```python
from build123d import *
from build123d.topology import SkipClean

# Parameters (mm, degrees)
SKETCH1_W               = 15
SKETCH1_H               = 23.93877551
BOSS_EXTRUDE1_DEPTH     = 25
CUT_EXTRUDE1_DEPTH      = 25
CUT_EXTRUDE2_DEPTH      = 33.787192622
CUT_EXTRUDE2_DEPTH_BACK = 33.787192622
SKETCH3_R               = 2.75
SKETCH4_W               = 9.5
SKETCH4_H               = 17
CUT_EXTRUDE3_DEPTH      = 8
CHAMFER1_SIZE           = 2
BOSS_EXTRUDE2_DEPTH     = 12.7
CHAMFER2_START          = 15.513056934
CHAMFER2_OUTLINE_W      = 15
CHAMFER2_OUTLINE_H      = 24
CHAMFER2_DEPTH          = 11.486943066


with BuildPart() as part:
    # Sketch1 → Boss-Extrude1 (new body)
    with BuildSketch(Plane.XY):
        with Locations((7.5, 11.969387755)):
            Rectangle(SKETCH1_W, SKETCH1_H)
    extrude(amount=BOSS_EXTRUDE1_DEPTH)

    # Sketch2 → Cut-Extrude1 (cut)
    with BuildSketch(Plane.XY.offset(25)):
        with BuildLine():
            Line((0, 8.93877551), (0, 0))
            Line((0, 0), (15, 0))
            Line((15, 0), (15, 8.93877551))
            ThreePointArc((15, 8.93877551), (7.5, 9.487151408), (0, 8.93877551))
        make_face()
    extrude(amount=-CUT_EXTRUDE1_DEPTH, mode=Mode.SUBTRACT)

    # Sketch3 → Cut-Extrude2 (cut, two sides: drawn at the far end of the back side and taken through both)
    with BuildSketch(Plane(origin=(0, 23.93877551, 0), x_dir=(1, 0, 0), z_dir=(0, 1, 0)).offset(-CUT_EXTRUDE2_DEPTH_BACK)):
        with Locations(Location((7.5, -8.825, 0), (0, 0, 270))):
            Circle(SKETCH3_R)
        with Locations(Location((7.5, -16.175, 0), (0, 0, 270))):
            Circle(SKETCH3_R)
    extrude(amount=CUT_EXTRUDE2_DEPTH + CUT_EXTRUDE2_DEPTH_BACK, mode=Mode.SUBTRACT)

    # Sketch4 → Cut-Extrude3 (cut)
    with BuildSketch(Plane(origin=(0, 23.93877551, 0), x_dir=(1, 0, 0), z_dir=(0, 1, 0))):
        with Locations((7.5, -12.5)):
            Rectangle(SKETCH4_W, SKETCH4_H)
    extrude(amount=-CUT_EXTRUDE3_DEPTH, mode=Mode.SUBTRACT)

    # Chamfer1
    chamfer1_edges = [part.edges().sort_by_distance(p)[0] for p in [
        (2.75, 19.93877551, 4),
        (12.25, 19.93877551, 4),
    ]]
    chamfer(chamfer1_edges, length=CHAMFER1_SIZE)

    # Sketch5 → Boss-Extrude2 (add)
    with SkipClean():  # the faces are left unmerged after this step: merging them gives an invalid solid
        with BuildSketch(Plane(origin=(0, 0, 0), x_dir=(-1, 0, 0), z_dir=(0, 0, -1))):
            with BuildLine():
                Line((-15, 23.93877551), (0, 23.93877551))
                Line((0, 23.93877551), (0, 8.93877551))
                ThreePointArc((0, 8.93877551), (-7.5, 9.487151408), (-15, 8.93877551))
                Line((-15, 8.93877551), (-15, 23.93877551))
            make_face()
        extrude(amount=BOSS_EXTRUDE2_DEPTH)

    # Chamfer2: read off the stored shape, not the designer's step
    # Chamfer2 outline → Chamfer2 (cut)
    with BuildSketch(Plane(origin=(0, 0, 0), x_dir=(1, 0, 0), z_dir=(0, 0.707106781186544, -0.707106781186551)).offset(CHAMFER2_START)):
        with Locations((7.5, -8)):
            Rectangle(CHAMFER2_OUTLINE_W, CHAMFER2_OUTLINE_H)
    extrude(amount=CHAMFER2_DEPTH, mode=Mode.SUBTRACT)


solid = part.part
```
Check sheet for the modelled part. Datum: model origin and axes. Units: mm. A direction names the side the tool comes from. Coordinates: 2 decimals unless noted, no trailing zeros. Loops run counter-clockwise (first coordinate to the right, second up) from the corner with the lowest first, then second, coordinate; pieces in that order, holes last. Notation, with made-up numbers: M 32.5,-15 L 36.5,-15 A16 ccw 36.5,15 Z; hole C -29.75,77 d3. An arc over 180 degrees is marked long. Answer as a JSON object with one key per item and string values.
1. Release check for a two-part mould opening along X. For faces 1 (the flat face through (15, 16, 11)), 2 (the cylindrical face through (5.722, 9.457, 6.414)), 3 (the flat face through (7.4, 16.49, -5.45)), 4 (the flat face through (3.74, 19.99, 5.01)) record: pulls with the +X half, pulls with the -X half, needs draft (parallel to the pull), parting line crosses it, or undercut.
Outcome:
{"face 1": "pulls with the +X half", "face 2": "undercut", "face 3": "needs draft", "face 4": "undercut"}
2. Sectioned sample at A-A on x = 8. Record the cut outline in (y, z), and give its area (3 significant figures).
Outcome:
{"outline": "M 9.48,-12.45 L 23.94,2 L 23.94,4 L 15.94,4 L 15.94,6.12 L 9.48,6.12 Z; M 9.48,11.53 L 15.94,11.53 L 15.94,13.47 L 9.48,13.47 Z; M 9.48,18.88 L 15.94,18.88 L 15.94,21 L 23.94,21 L 23.94,25 L 9.48,25 Z", "area": "231 mm²"}
3. Access from +Z, -Z, +X, -X, +Y, -Y to the whole of each face (thin tool, end or side, straight path). Record for faces 5 (the flat face through (12.25, 20, 14)), 6 (the flat face through (0, 16, 10)).
Outcome:
{"face 5": "+Y", "face 6": "+Z, -Z, -X, +Y, -Y"}
4. Sectioned sample at B-B on z = 18. Record the cut outline in (x, y).
Outcome:
{"outline": "M 0,8.94 A51.56 cw 5.44,9.45 L 5.44,15.94 L 2.75,15.94 L 2.75,23.94 L 0,23.94 Z; M 9.56,9.45 A51.56 cw 15,8.94 L 15,23.94 L 12.25,23.94 L 12.25,15.94 L 9.56,15.94 Z"}
5. Depth check by flat-ended pin: P1, Ø3, axis at x = 5.5, y = 20, coming from the -Z side; P2, Ø6.5, axis at x = 8, y = 19, coming from the -Z side; P3, Ø2, axis at x = 1.5, z = 17.5, coming from the -Y side. Enter the tip coordinate at first touch or a pass-through.
Outcome:
{"P1": "z = -3.44", "P2": "z = -6.19", "P3": "y = 9.01"}
6. Scan lines: L1, parallel to X at y = 17.5, z = 12; L2, parallel to Z at x = 7.5, y = 13.75 (3 decimals); L3, parallel to Z at x = 9, y = 13. Record each from-to range of solid material in increasing order. Write a range as from..to.
Outcome:
{"L1": "0..2.75, 12.25..15", "L2": "-8.189..6.075, 11.575..13.425, 18.925..25", "L3": "-8.94..6.52, 11.13..13.87, 18.48..25"}
7. Sectioned sample at D-D on x = 3.25. Record the cut outline in (y, z), and give its area (3 significant figures).
Outcome:
{"outline": "M 9.31,-12.63 L 23.94,2 L 23.94,5.5 L 15.94,5.5 L 15.94,21 L 23.94,21 L 23.94,25 L 9.31,25 Z", "area": "319 mm²"}
8. Sectioned sample at C-C on y = 19.75. Record the cut outline in (x, z).
Outcome:
{"outline": "M 0,-2.19 L 15,-2.19 L 15,25 L 0,25 Z; hole M 2.75,6 L 4.75,4 L 10.25,4 L 12.25,6 L 12.25,21 L 2.75,21 Z"}
